Here's how the part is built. I have some questions about the finished solid (model axes, mm). A direction names the side the tool comes from. Coordinates: 2 decimals unless noted, no trailing zeros. Loops run counter-clockwise (first coordinate to the right, second up) from the corner with the lowest first, then second, coordinate; pieces in that order, holes last. Notation, with made-up numbers: M 40.25,34 L 54.25,34 A17 cw 54.25,53 Z; hole C -26.75,-34.75 d6. An arc over 180 degrees is marked long. Use one line per item in the form item = value. Start each with the question number.
(1) Please list where these lines run through material, in increasing order: L1, parallel to X at y = -2, z = -19.05 (3 decimals); L2, parallel to Y at x = -50.5, z = -33 (3 decimals); L3, parallel to Z at x = 17.5, y = 2.5.
(2) Thinking about a two-plate mould opening in X: for faces 6 (the flat face through (-12.06, 1.5, -22.73)), 7 (the flat face through (-2, 1, 29.726)), 8 (the flat face through (-1.535, 1.545, -13.729)), which applies, +X half, -X half, draft (parallel to the pull), parting line (faces both ways), or undercut?
(3) Will these pins go through, and if not, where does the flat tip stop? P1, Ø2, axis at y = 2, z = -12, coming from the +X side; P2, Ø0.9, axis at x = -11.5, y = 2, coming from the +Z side; P3, Ø0.6, axis at x = 56.5, y = -1, coming from the +Z side; P4, Ø2, axis at x = -56.515, z = 19.05, coming from the -Y side.
(4) On a 3-axis mill with a long thin cutter (end or side, diameter ignored), from which of +Z, -Z, +X, -X, +Y, -Y can I reach the whole of each face in a straight line? I mean faces 1 (the flat face through (-3.06, 1.5, -4.73)), 2 (the flat face through (16.62, 1, 13)), 3 (the flat face through (21.17, 1.55, 32)), 4 (the flat face through (-2, 1, 23.774)), 5 (the flat face through (12.03, 1.55, -22)). Say none if no direction works.
(5) Imagine slicing it at A-A, the plane z = 19.05. Please give me the cut outline in (x, y) (3 decimals), and give its area (3 significant figures).
(6) Imagine slicing it at C-C, the plane x = -43. Please give me the cut outline in (y, z) (3 decimals).
(7) Imagine slicing it at B-B, the plane y = -1.5. Please give me the cut outline in (x, z) (3 decimals).
```python
from build123d import *

# Parameters (mm, degrees)
SKETCH1_W            = 109.22
SKETCH1_H            = 73.66
BOSS_EXTRUDE1_DEPTH  = 3.175
BOSS_EXTRUDE3_DEPTH  = 1.524
LPATTERN1_COUNT      = 2
LPATTERN1_PITCH      = 9.000000034
LPATTERN1_COUNT_DIR2 = 8
LPATTERN1_PITCH_DIR2 = 9.000000034
SKETCH3_W            = 3.81
SKETCH3_H            = 50.8
SKETCH3_R            = 1.27
BOSS_EXTRUDE2_DEPTH  = 3.175
FILLET1_R            = 1.651
BOSS_EXTRUDE4_START  = 8.999982
BOSS_EXTRUDE4_DEPTH  = 3.048
BOSS_EXTRUDE5_START  = 10.523982
BOSS_EXTRUDE5_DEPTH  = 3.048
BOSS_EXTRUDE6_START  = 12.047982
BOSS_EXTRUDE6_DEPTH  = 3.048
BOSS_EXTRUDE7_START  = 13.571982
BOSS_EXTRUDE7_DEPTH  = 3.048
BOSS_EXTRUDE8_START  = 15.095982
BOSS_EXTRUDE8_DEPTH  = 3.048
BOSS_EXTRUDE9_START  = 16.619982
BOSS_EXTRUDE9_DEPTH  = 3.048
BOSS_EXTRUDE10_START = 18.143982
BOSS_EXTRUDE10_DEPTH = 3.048
BOSS_EXTRUDE11_START = 19.667982
BOSS_EXTRUDE11_DEPTH = 3.048


with BuildPart() as part:
    # Sketch1 → Boss-Extrude1 (new body)
    with BuildSketch(Plane(origin=(0, 0, 0), x_dir=(1, 0, 0), z_dir=(0, 1, 0))):
        Rectangle(SKETCH1_W, SKETCH1_H)
    extrude(amount=-BOSS_EXTRUDE1_DEPTH)

    # Sketch2 → Boss-Extrude3 (add, symmetric)
    with BuildSketch(Plane.XY.offset(-31.75)):
        Polygon((-12.810000034, 0), (-11.286000034, 3.048), (-9.762000034, 0), (-11.286000034, 0), align=None)
    boss_extrude3 = extrude(amount=BOSS_EXTRUDE3_DEPTH, both=True)

    # LPattern1: Boss-Extrude3 2 × 8
    with Locations(*[(i * LPATTERN1_PITCH, 0, j * LPATTERN1_PITCH_DIR2) for i in range(LPATTERN1_COUNT) for j in range(LPATTERN1_COUNT_DIR2) if (i, j) != (0, 0)]):
        add(boss_extrude3)

    # Sketch3 → Boss-Extrude2 (add)
    # profile 1 of 2: a face of its own
    with BuildSketch(Plane(origin=(0, 0, 0), x_dir=(1, 0, 0), z_dir=(0, 1, 0))):
        with Locations((-56.515, 0)):
            Rectangle(SKETCH3_W, SKETCH3_H)
        with Locations(Location((-56.515, 19.05, 0), (0, 0, 270))):
            Circle(SKETCH3_R, mode=Mode.SUBTRACT)
        with Locations(Location((-56.515, -19.05, 0), (0, 0, 270))):
            Circle(SKETCH3_R, mode=Mode.SUBTRACT)
    # profile 2 of 2: a face of its own
    with BuildSketch(Plane(origin=(0, 0, 0), x_dir=(1, 0, 0), z_dir=(0, 1, 0))):
        with Locations((56.515, 0)):
            Rectangle(SKETCH3_W, SKETCH3_H)
        with Locations(Location((56.515, -19.05, 0), (0, 0, 90))):
            Circle(SKETCH3_R, mode=Mode.SUBTRACT)
        with Locations(Location((56.515, 19.05, 0), (0, 0, 90))):
            Circle(SKETCH3_R, mode=Mode.SUBTRACT)
    extrude(amount=-BOSS_EXTRUDE2_DEPTH)

    # Fillet1
    fillet1_edges = [part.edges().sort_by_distance(p)[0] for p in [
        (-54.61, -1.5875, -25.4),
        (-54.61, -1.5875, 25.4),
        (-58.42, -1.5875, 25.4),
        (-58.42, -1.5875, -25.4),
        (54.61, -1.5875, -25.4),
        (58.42, -1.5875, -25.4),
        (58.42, -1.5875, 25.4),
        (54.61, -1.5875, 25.4),
        (54.61, -1.5875, 36.83),
        (-54.61, -1.5875, 36.83),
        (-54.61, -1.5875, -36.83),
        (54.61, -1.5875, -36.83),
    ]]
    fillet(fillet1_edges, radius=FILLET1_R)

    # Sketch4 → Boss-Extrude4 (add)
    with BuildSketch(Plane(origin=(0, 0, 0), x_dir=(0, 0, -1), z_dir=(1, 0, 0)).offset(BOSS_EXTRUDE4_START)):
        Polygon((30.226, 0), (33.274, 0), (31.75, 3.048), align=None)
    extrude(amount=BOSS_EXTRUDE4_DEPTH)

    # Sketch5 → Boss-Extrude5 (add)
    with BuildSketch(Plane(origin=(0, 0, 0), x_dir=(0, 0, -1), z_dir=(1, 0, 0)).offset(BOSS_EXTRUDE5_START)):
        Polygon((21.225999966, 0), (24.273999966, 0), (22.749999966, 3.048), align=None)
    extrude(amount=BOSS_EXTRUDE5_DEPTH)

    # Sketch6 → Boss-Extrude6 (add)
    with BuildSketch(Plane(origin=(0, 0, 0), x_dir=(0, 0, -1), z_dir=(1, 0, 0)).offset(BOSS_EXTRUDE6_START)):
        Polygon((12.225999932, 0), (15.273999932, 0), (13.749999932, 3.048), align=None)
    extrude(amount=BOSS_EXTRUDE6_DEPTH)

    # Sketch7 → Boss-Extrude7 (add)
    with BuildSketch(Plane(origin=(0, 0, 0), x_dir=(0, 0, -1), z_dir=(1, 0, 0)).offset(BOSS_EXTRUDE7_START)):
        Polygon((3.225999898, 0), (6.273999898, 0), (4.749999898, 3.048), align=None)
    extrude(amount=BOSS_EXTRUDE7_DEPTH)

    # Sketch8 → Boss-Extrude8 (add)
    with BuildSketch(Plane(origin=(0, 0, 0), x_dir=(0, 0, -1), z_dir=(1, 0, 0)).offset(BOSS_EXTRUDE8_START)):
        Polygon((-5.774000136, 0), (-2.726000136, 0), (-4.250000136, 3.048), align=None)
    extrude(amount=BOSS_EXTRUDE8_DEPTH)

    # Sketch9 → Boss-Extrude9 (add)
    with BuildSketch(Plane(origin=(0, 0, 0), x_dir=(0, 0, -1), z_dir=(1, 0, 0)).offset(BOSS_EXTRUDE9_START)):
        Polygon((-14.77400017, 0), (-11.72600017, 0), (-13.25000017, 3.048), align=None)
    extrude(amount=BOSS_EXTRUDE9_DEPTH)

    # Sketch10 → Boss-Extrude10 (add)
    with BuildSketch(Plane(origin=(0, 0, 0), x_dir=(0, 0, -1), z_dir=(1, 0, 0)).offset(BOSS_EXTRUDE10_START)):
        Polygon((-23.774000204, 0), (-20.726000204, 0), (-22.250000204, 3.048), align=None)
    extrude(amount=BOSS_EXTRUDE10_DEPTH)

    # Sketch11 → Boss-Extrude11 (add)
    with BuildSketch(Plane(origin=(0, 0, 0), x_dir=(0, 0, -1), z_dir=(1, 0, 0)).offset(BOSS_EXTRUDE11_START)):
        Polygon((-32.774000238, 0), (-29.726000238, 0), (-31.250000238, 3.048), align=None)
    extrude(amount=BOSS_EXTRUDE11_DEPTH)


solid = part.part
```
Answer:
q1.L1 = -58.42 to -57.785, -55.245 to 55.245, 57.785 to 58.42
q1.L2 = -3.175 to 0
q1.L3 = 3.98 to 4.52, 12.98 to 13.52
q2.face_6 = -X half
q2.face_7 = draft
q2.face_8 = undercut
q3.P1 = -1.27
q3.P2 = 32.77
q3.P3 = 25.4
q3.P4 = through
q4.face_1 = +Z, -Z, +Y
q4.face_2 = +Z, +Y
q4.face_3 = +Z, +X, +Y
q4.face_4 = +X, -X, +Y
q4.face_5 = +X, +Y
q5.outline = M -58.42,-3.175 L -57.785,-3.175 L -57.785,0 L -58.42,0 Z; M -55.245,-3.175 L 55.245,-3.175 L 55.245,0 L -55.245,0 Z; M 57.785,-3.175 L 58.42,-3.175 L 58.42,0 L 57.785,0 Z
q5.area = 355 mm²
q6.outline = M -3.175,-36.83 L 0,-36.83 L 0,36.83 L -3.175,36.83 Z
q7.outline = M -58.42,-23.749 A1.651 ccw -56.769,-25.4 L -56.261,-25.4 A1.651 cw -54.61,-27.051 L -54.61,-35.179 A1.651 ccw -52.959,-36.83 L 52.959,-36.83 A1.651 ccw 54.61,-35.179 L 54.61,-27.051 A1.651 cw 56.261,-25.4 L 56.769,-25.4 A1.651 ccw 58.42,-23.749 L 58.42,23.749 A1.651 ccw 56.769,25.4 L 56.261,25.4 A1.651 cw 54.61,27.051 L 54.61,35.179 A1.651 ccw 52.959,36.83 L -52.959,36.83 A1.651 ccw -54.61,35.179 L -54.61,27.051 A1.651 cw -56.261,25.4 L -56.769,25.4 A1.651 ccw -58.42,23.749 Z; hole C -56.515,-19.05 d2.54; hole C -56.515,19.05 d2.54; hole C 56.515,-19.05 d2.54; hole C 56.515,19.05 d2.54
